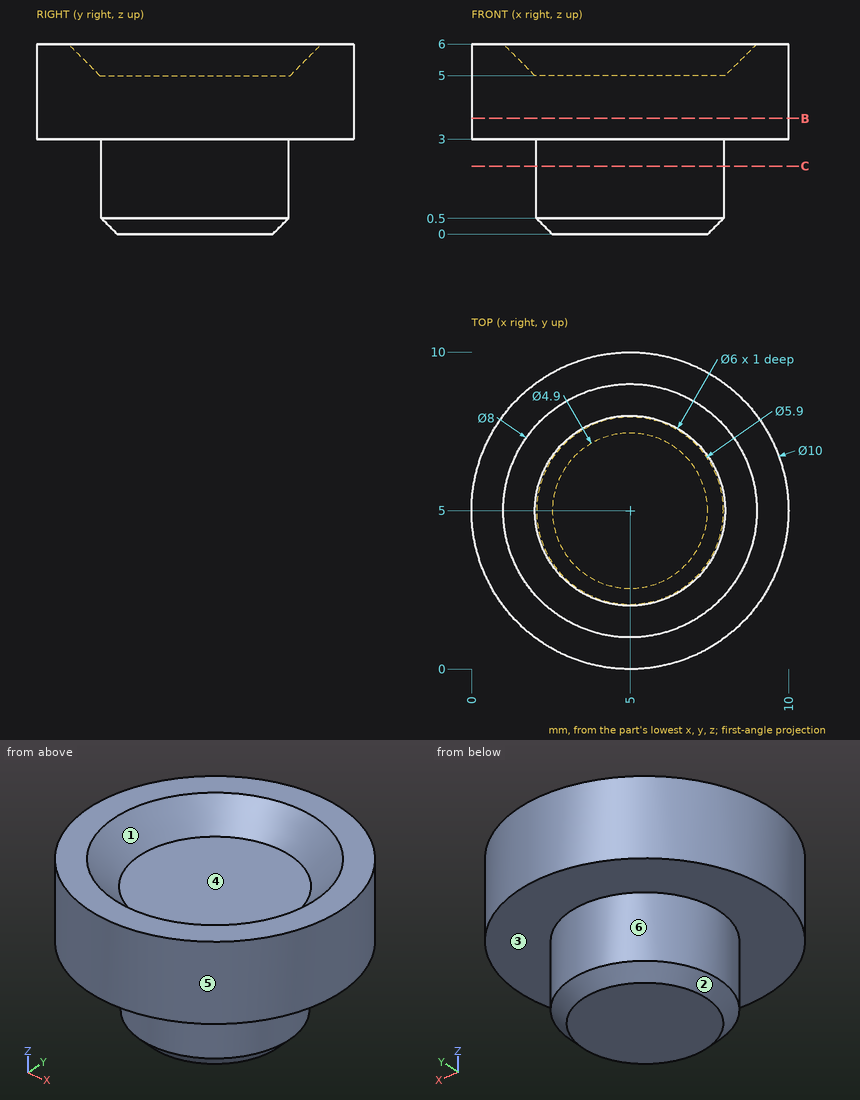
Check sheet for the drawn part. Datum: minimum x, y, z corner. Units: mm. A direction names the side the tool comes from. Give positions to 0.01 mm unless a question says otherwise; leave off trailing zeros. Order: outer loops, then holes, each group sorted by start corner. A loop starts at its lowest first (then second) coordinate and runs counter-clockwise, first axis right, second up. Notation, with made-up numbers: (9, 60.25) - (39, 60.25) arc R22 cw to (39, 73.25) - close; hole circle Ø9 at (26, 21). An arc over 180 degrees is marked (long way). Answer as a JSON object with one key per item and string values.
(1) Draft check along X on the marked faces 1, 2 and 3. Enter one of: released by +X, released by -X, zero draft, split by the parting line, or undercut.
Report:
{"face 1": "undercut", "face 2": "split by the parting line", "face 3": "zero draft"}
(2) Cross-section at C-C (z = 2.15). Record the cut outline in (x, y).
Report:
{"outline": "circle Ø5.9 at (5, 5)"}
(3) Depth check by flat-ended pin: pin 1 Ø3 at (x, z) = (3, 4.5) entering from -Y (3 decimals); pin 2 Ø3 at (x, y) = (5, 7) entering from +Z; pin 3 Ø1.8 at (x, y) = (3.5, 4.5) entering from +Z. Enter the tip coordinate at first touch or a pass-through.
Report:
{"pin 1": "y = 0.025", "pin 2": "z = 5.5", "pin 3": "z = 5"}
(4) Cross-section at B-B (z = 3.65). Record the cut outline in (x, y).
Report:
{"outline": "circle Ø10 at (5, 5)"}
(5) Material ranges on line 1 (Z direction, x = 3, y = 5); line 2 (Z direction, x = 7.25, y = 1.25); line 3 (Y direction, x = 5, z = 5.05), recorded low to high.
Report:
{"line 1": "0 to 5", "line 2": "3 to 6", "line 3": "0 to 1.95, 8.05 to 10"}
(6) Tool access check on the marked faces 4, 5 and 6. Record the directions out of +Z, -Z, +X, -X, +Y, -Y that give a thin tool (end or side, any length) a straight path to the whole face; none if there is none.
Report:
{"face 4": "+Z", "face 5": "+Z, -Z", "face 6": "-Z"}
